Can you work these out from the model? Positions are in its coordinate system, mm. A direction names the side the tool comes from. Give positions to 0.01 mm unless a question says otherwise; leave off trailing zeros. Loops run counter-clockwise (first coordinate to the right, second up) from the corner with the lowest first, then second, coordinate; pieces in that order, holes last. Notation, with made-up numbers: (-2, -13.5) - (22, -13.5) arc R23 ccw to (22, 23.5) - close; hole circle Ø11 at (75.25, 70). An arc over 180 degrees is marked (long way). Answer in a Markdown table with one row per item.
from build123d import *

# Parameters (mm, degrees)
SKETCH_1_W          = 10
SKETCH_1_H          = 10
SKETCH_1_W_2        = 8
SKETCH_1_H_2        = 8
EXTRUDE_1_DEPTH     = 150
SKETCH_2_R          = 1.5
CUT_EXTRUDE_1_DEPTH = 11
SKETCH_3_R          = 1.5
CUT_EXTRUDE_2_DEPTH = 11


with BuildPart() as part:
    # 草图1 → 拉伸-薄壁1 (new body)
    with BuildSketch(Plane.XY):
        with Locations((211.703793946, 99.48732034)):
            Rectangle(SKETCH_1_W, SKETCH_1_H)
        with Locations((211.703793946, 99.48732034)):
            Rectangle(SKETCH_1_W_2, SKETCH_1_H_2, mode=Mode.SUBTRACT)
    extrude(amount=EXTRUDE_1_DEPTH)

    # 草图2 → 切除-拉伸1 (cut, through all)
    with BuildSketch(Plane(origin=(216.703793946, 0, 0), x_dir=(0, 0, -1), z_dir=(1, 0, 0))):
        with Locations((-30, 99.48732034)):
            Circle(SKETCH_2_R)
        with Locations((-5, 99.48732034)):
            Circle(SKETCH_2_R)
        with Locations((-130, 99.48732034)):
            Circle(SKETCH_2_R)
        with Locations((-140, 99.48732034)):
            Circle(SKETCH_2_R)
    extrude(amount=-CUT_EXTRUDE_1_DEPTH, mode=Mode.SUBTRACT)

    # 草图3 → 切除-拉伸2 (cut, through all)
    with BuildSketch(Plane.XZ.offset(-94.48732034)):
        with Locations((211.703793946, 120)):
            Circle(SKETCH_3_R)
        with Locations((211.703793946, 35)):
            Circle(SKETCH_3_R)
        with Locations((211.703793946, 145)):
            Circle(SKETCH_3_R)
        with Locations((211.703793946, 60)):
            Circle(SKETCH_3_R)
        with Locations((211.703793946, 15)):
            Circle(SKETCH_3_R)
    extrude(amount=-CUT_EXTRUDE_2_DEPTH, mode=Mode.SUBTRACT)


solid = part.part
Q1. If I drill on line 1 (Y direction, x = 216.5, z = 5); line 2 (Y direction, x = 212, z = 117); line 3 (X direction, y = 102.5, z = 23.5), over which ranges is the centre line in solid material (lowest first)? Write a range as [from, to].
Checked values:
| item | result |
|---|---|
| line 1 | y = [94.49, 97.99], [100.99, 104.49] |
| line 2 | y = [94.49, 95.49], [103.49, 104.49] |
| line 3 | x = [206.7, 207.7], [215.7, 216.7] |
Q2. If we mould it in two halves opening along Y, with no side actions, what happens to faces 3 (the face through (207.704, 99, 74)), 4 (the face through (210.205, 94.98, 15.066)), 5 (the face through (212, 104.487, 74))? For each: released by +Y, released by -Y, zero draft, split by the parting line, or undercut.
Checked values:
| item | result |
|---|---|
| face 3 | undercut |
| face 4 | zero draft |
| face 5 | released by +Y |
Q3. On a 3-axis mill with a long thin cutter (end or side, diameter ignored), from which of +Z, -Z, +X, -X, +Y, -Y can I reach the whole of each face in a straight line? I mean faces 1 (the face through (212, 95.487, 74)), 2 (the face through (210.598, 94.98, 61.014)). Say none if no direction works.
Checked values:
| item | result |
|---|---|
| face 1 | +Z, -Z |
| face 2 | +Y, -Y |
Q4. Imagine slicing it at C-C, the plane z = 96. Write out the boundary of the cut face in (x, y).
Checked values:
| item | result |
|---|---|
| outline | (206.7, 94.49) - (216.7, 94.49) - (216.7, 104.49) - (206.7, 104.49) - close; hole (207.7, 95.49) - (215.7, 95.49) - (215.7, 103.49) - (207.7, 103.49) - close |
Q5. Imagine slicing it at A-A, the plane z = 120. Write out the boundary of the cut face in (x, y), and give its area (3 significant figures).
Checked values:
| item | result |
|---|---|
| outline | (206.7, 94.49) - (210.2, 94.49) - (210.2, 95.49) - (207.7, 95.49) - (207.7, 103.49) - (210.2, 103.49) - (210.2, 104.49) - (206.7, 104.49) - close; (213.2, 94.49) - (216.7, 94.49) - (216.7, 104.49) - (213.2, 104.49) - (213.2, 103.49) - (215.7, 103.49) - (215.7, 95.49) - (213.2, 95.49) - close |
| area | 30.0 mm² |
Q6. Imagine slicing it at B-B, the plane y = 102.25. Write out the boundary of the cut face in (x, z), and give its area (3 significant figures).
Checked values:
| item | result |
|---|---|
| outline | (206.7, 0) - (207.7, 0) - (207.7, 150) - (206.7, 150) - close; (215.7, 0) - (216.7, 0) - (216.7, 150) - (215.7, 150) - close |
| area | 300 mm² |
Q7. For pin 1 (1.8 mm diameter, centred on x = 211.7, z = 35, fed in from -Y) (3 decimals), with a flat end and sliding along its axis, tell me the tip position at first contact or that it passes through.
Checked values:
| item | result |
|---|---|
| pin 1 | passes through |
